```python
from build123d import *

# Parameters (mm, degrees)
F0_W     = 105
F0_H     = 40
F1_DEPTH = 15
F3_D     = 4
F3_DEPTH = 12
F3_TIP   = 1.2017212381
F5_D     = 4
F5_DEPTH = 12
F5_TIP   = 1.2017212381


with BuildPart() as f1:
    # F0 (on Right) → F1 (new body)
    with BuildSketch(Plane.YZ):
        Rectangle(F0_W, F0_H)
    extrude(amount=F1_DEPTH)

    # F3
    with Locations(Plane.XZ.offset(52.5)):
        with Locations((7.5, 0)):
            Hole(F3_D / 2, depth=F3_DEPTH)
            with Locations((0, 0, -(F3_DEPTH + F3_TIP / 2))):  # 118° drill point
                Cone(0, F3_D / 2, F3_TIP, mode=Mode.SUBTRACT)

    # F5
    with Locations(Plane(origin=(0, 0, -20), x_dir=(1, 0, 0), z_dir=(0, 0, -1))):
        with Locations((7.5, 45), (7.5, -45)):
            Hole(F5_D / 2, depth=F5_DEPTH)
            with Locations((0, 0, -(F5_DEPTH + F5_TIP / 2))):  # 118° drill point
                Cone(0, F5_D / 2, F5_TIP, mode=Mode.SUBTRACT)


solid = f1.part
```
The listing builds one solid part. Answer for the finished solid, in the listing's coordinates (mm). A direction names the side the tool comes from. Give positions to 0.01 mm unless a question says otherwise; leave off trailing zeros. Write each question's results on one line, items separated by ' | '.
Q1. A tool of negligible diameter and unlimited length cuts with its end or side. For faces 1 (the flat face through (7, 52.5, 0)), 2 (the cylindrical face through (9.498, -46.416, 0.088)), 3 (the cylindrical face through (7.934, -43.048, -13.916)), from which of +Z, -Z, +X, -X, +Y, -Y can it reach the whole face along a straight path? Write none if from no direction.
Output values:
face 1: +Z, -Z, +X, -X, +Y | face 2: -Y | face 3: -Z
Q2. Consider L1, parallel to Y at x = 7.5, z = -16.5; L2, parallel to Y at x = 9.25, z = -14; L3, parallel to X at y = -45, z = -15. Determine where each line is inside the solid, lowest interval first. Write a range as from..to.
Output values:
L1: -52.5..-47, -43..43, 47..52.5 | L2: -52.5..-45.97, -44.03..44.03, 45.97..52.5 | L3: 0..5.5, 9.5..15
Q3. For a pull along X with two mould halves and no side action, classify faces 4 (the flat face through (4, -52.5, 0)), 5 (the conical face through (7.42, -44.66, -7.01)), 6 (the flat face through (0, -1, 0)), 7 (the flat face through (15, -1, 0)) as released by +X, released by -X, zero draft, split by the parting line, or undercut.
Output values:
face 4: zero draft | face 5: undercut | face 6: released by -X | face 7: released by +X
